Part model, mm, in its own coordinate system. Face numbers are marked on the shaded views. A direction names the side the tool comes from. Round coordinates to 2 decimals unless told otherwise and drop trailing zeros. Write each loop counter-clockwise with the first axis right and the second up, starting at its lowest first coordinate (ties: lowest second). Pieces come first, ordered by that corner, then holes. Notation, with made-up numbers: M 73.5,32 L 110.5,32 A17 cw 110.5,39 Z; hole C 2,31.5 d7. An arc over 180 degrees is marked long. Answer as a JSON object with one key per item and string values. Group by question number.
1. Which spindle directions (+Z, -Z, +X, -X, +Y, -Y) get a long thin tool onto all of the face, cutting with end or side? Do the marked faces 4 and 5. Say none if no direction does.
2. Drop flat-ended pins along their axis: pin 1 (8 mm diameter, centred on y = 8.5, z = -1.5, fed in from +X); pin 2 (4 mm diameter, centred on x = 1, z = -0.5, fed in from +Y); pin 3 (6 mm diameter, centred on x = 6, z = 5, fed in from -Y); pin 4 (1 mm diameter, centred on x = 5.5, y = 14, fed in from +Z). Give the stop position or say it passes through.
3. Band-saw the part on D-D, the plane x = 8. Write the cut outline in (y, z), plus the area to 3 significant figures.
4. Two-plate mould, pull along Z, no slides. Class the marked faces 1, 2 and 3: +Z half, -Z half, draft (parallel to the pull), parting line (faces both ways), or undercut.
5. Drill centre lines: line 1 (Y direction, x = 6, z = 0); line 2 (Y direction, x = -6.75, z = 4.75); line 3 (Y direction, x = 2.25, z = -1.5). Where is each one in solid material? Low to high. Write a range as from..to.
6. Band-saw the part on A-A, the plane x = 6. Write the cut outline in (y, z).
7. Band-saw the part on C-C, the plane z = -4.5. Write the cut outline in (x, y).
8. Band-saw the part on B-B, the plane x = 0. Write the cut outline in (y, z), plus the area to 3 significant figures.
from build123d import *

# Parameters (mm, degrees)
SKETCH1_R           = 7.5
SKETCH1_R_2         = 2.5
BOSS_EXTRUDE1_DEPTH = 22
SKETCH2_R           = 7.5
BOSS_EXTRUDE2_DEPTH = 8
SKETCH3_R           = 9.5
BOSS_EXTRUDE3_DEPTH = 20
SKETCH5_R           = 4
CUT_EXTRUDE1_DEPTH  = 15
SKETCH6_R           = 2
CUT_EXTRUDE2_DEPTH  = 17


with BuildPart() as part:
    # Sketch1 → Boss-Extrude1 (new body)
    with BuildSketch(Plane(origin=(0, 0, 0), x_dir=(1, 0, 0), z_dir=(0, 1, 0))):
        with Locations(Location((0, 0, 0), (0, 0, 270))):
            Circle(SKETCH1_R)
        with Locations(Location((0, 0, 0), (0, 0, 270))):
            Circle(SKETCH1_R_2, mode=Mode.SUBTRACT)
    extrude(amount=BOSS_EXTRUDE1_DEPTH)

    # Sketch2 → Boss-Extrude2 (add)
    with BuildSketch(Plane(origin=(0, 22, 0), x_dir=(1, 0, 0), z_dir=(0, 1, 0))):
        with Locations(Location((0, 0, 0), (0, 0, 270))):
            Circle(SKETCH2_R)
    extrude(amount=BOSS_EXTRUDE2_DEPTH)

    # Sketch3 → Boss-Extrude3 (add)
    with BuildSketch(Plane(origin=(0, 30, 0), x_dir=(1, 0, 0), z_dir=(0, 1, 0))):
        with Locations(Location((0, 0, 0), (0, 0, 270))):
            Circle(SKETCH3_R)
    extrude(amount=BOSS_EXTRUDE3_DEPTH)

    # Sketch5 → Cut-Extrude1 (cut)
    with BuildSketch(Plane(origin=(0, 50, 0), x_dir=(1, 0, 0), z_dir=(0, 1, 0))):
        with Locations(Location((0, 0, 0), (0, 0, 270))):
            Circle(SKETCH5_R)
    extrude(amount=-CUT_EXTRUDE1_DEPTH, mode=Mode.SUBTRACT)

    # Sketch6 → Cut-Extrude2 (cut)
    with BuildSketch(Plane(origin=(0, 0, 0), x_dir=(0, 0, -1), z_dir=(1, 0, 0))):
        with Locations(Location((0, 15, 0), (0, 0, 180))):
            Circle(SKETCH6_R)
        with Locations(Location((0, 40, 0), (0, 0, 180))):
            Circle(SKETCH6_R)
    extrude(amount=CUT_EXTRUDE2_DEPTH, mode=Mode.SUBTRACT)


solid = part.part
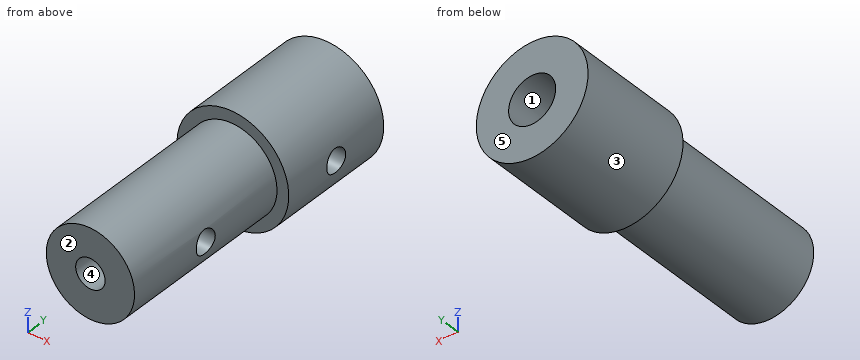
Worked answers:
{
 "1": {"face 4": "-Y", "face 5": "+Z, -Z, +X, -X, +Y"},
 "2": {"pin 1": "stops at x = 7.5", "pin 2": "stops at y = 35", "pin 3": "stops at y = 0", "pin 4": "stops at z = 5.59"},
 "3": {"outline": "M 30,-5.12 L 50,-5.12 L 50,5.12 L 30,5.12 Z; hole C 40,0 d4", "area": "192 mm^2"},
 "4": {"face 1": "undercut", "face 2": "draft", "face 3": "parting line"},
 "5": {"line 1": "y = 0..13, 17..38, 42..50", "line 2": "y = 30..50", "line 3": "y = 0..13.68, 16.32..35"},
 "6": {"outline": "M 0,-4.5 L 30,-4.5 L 30,-7.37 L 50,-7.37 L 50,7.37 L 30,7.37 L 30,4.5 L 0,4.5 Z; hole C 15,0 d4; hole C 40,0 d4"},
 "7": {"outline": "M -8.37,30 L -6,30 L -6,0 L 6,0 L 6,30 L 8.37,30 L 8.37,50 L -8.37,50 Z"},
 "8": {"outline": "M 0,-7.5 L 30,-7.5 L 30,-9.5 L 50,-9.5 L 50,-4 L 35,-4 L 35,4 L 50,4 L 50,9.5 L 30,9.5 L 30,7.5 L 0,7.5 L 0,2.5 L 22,2.5 L 22,-2.5 L 0,-2.5 Z", "area": "600 mm^2"}
}
